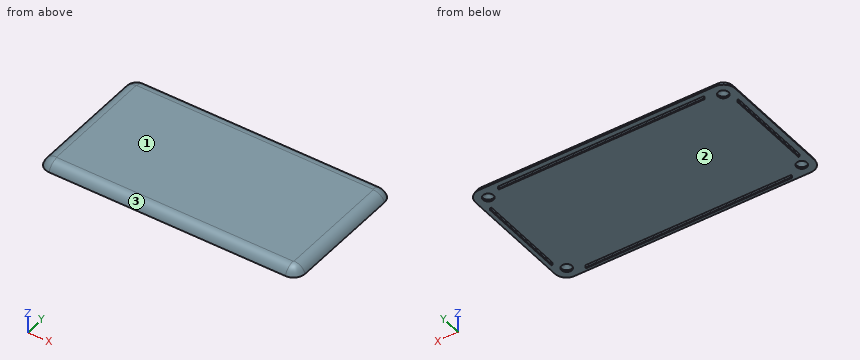
from build123d import *

# Parameters (mm, degrees)
F1_DEPTH     = 3.5
F5_D         = 4.473
F5_DEPTH     = 0.8
F5_TIP       = 1.3438247745
F6_T1_DEPTH  = 101
F6_T3_DEPTH  = 48.5
F6_T6_ANGLE  = 90
F6_T8_ANGLE  = 90
F6_T10_ANGLE = 90
F6_T12_ANGLE = 90
F8_W         = 0.5
F8_H         = 37.5
F8_W_2       = 88
F8_H_2       = 0.5
F9_DEPTH     = 1


# Not quite as in the source:
# - a fillet or chamfer that OpenCascade refuses, or shapes differently, is made with other operations: its cross-section is extruded or revolved along the edge and cut away or added


with BuildPart() as f1:
    # F0 (on Top) → F1 (new body)
    with BuildSketch(Plane.XY):
        with BuildLine():
            Line((-50.5, -29.25), (50.5, -29.25))
            ThreePointArc((50.5, -29.25), (54.0355339059, -27.7855339059), (55.5, -24.25))
            Line((55.5, -24.25), (55.5, 24.25))
            ThreePointArc((55.5, 24.25), (54.0355339059, 27.7855339059), (50.5, 29.25))
            Line((50.5, 29.25), (-50.5, 29.25))
            ThreePointArc((-50.5, 29.25), (-54.0355339059, 27.7855339059), (-55.5, 24.25))
            Line((-55.5, 24.25), (-55.5, -24.25))
            ThreePointArc((-55.5, -24.25), (-54.0355339059, -27.7855339059), (-50.5, -29.25))
        make_face()
    extrude(amount=F1_DEPTH)

    # F5
    with Locations(Plane(origin=(0, 0, 0), x_dir=(1, 0, 0), z_dir=(0, 0, -1))):
        with Locations((-50.2406740561, -23.9985361695), (-50.2495961264, 24.0030474961), (50.2488752827, 23.995583877), (50.2413948998, -24.0000952035)):
            Hole(F5_D / 2, depth=F5_DEPTH)
            with Locations((0, 0, -(F5_DEPTH + F5_TIP / 2))):  # 118° drill point
                Cone(0, F5_D / 2, F5_TIP, mode=Mode.SUBTRACT)

    # F6: fillet of radius 5 on 1 edges, made by hand

    # F6_s2 → F6_t1 (cut)
    with BuildSketch(Plane.YZ.offset(-50.5)):
        with BuildLine():
            ThreePointArc((-29.25, 0), (-27.4383438845, 2.5311288741), (-24.4803039929, 3.5))
            Line((-24.4803039929, 3.5), (-29.25, 3.5))
            Line((-29.25, 3.5), (-29.25, 0))
        make_face()
        with BuildLine():
            ThreePointArc((24.4803039929, 3.5), (27.4383438845, 2.5311288741), (29.25, 0))
            Line((29.25, 0), (29.25, 3.5))
            Line((29.25, 3.5), (24.4803039929, 3.5))
        make_face()
    extrude(amount=F6_T1_DEPTH, mode=Mode.SUBTRACT)

    # F6_s4 → F6_t3 (cut)
    with BuildSketch(Plane.XZ.offset(-24.25)):
        with BuildLine():
            ThreePointArc((50.7303039929, 3.5), (53.6883438845, 2.5311288741), (55.5, 0))
            Line((55.5, 0), (55.5, 3.5))
            Line((55.5, 3.5), (50.7303039929, 3.5))
        make_face()
        with BuildLine():
            ThreePointArc((-50.7303039929, 3.5), (-53.6883438845, 2.5311288741), (-55.5, 0))
            Line((-55.5, 0), (-55.5, 3.5))
            Line((-55.5, 3.5), (-50.7303039929, 3.5))
        make_face()
    extrude(amount=F6_T3_DEPTH, mode=Mode.SUBTRACT)

    # F6_s5 → F6_t6 (revolve, cut)
    with BuildSketch(Plane.XZ.offset(24.25)):
        with BuildLine():
            ThreePointArc((-55.5, 0), (-53.6883438845, 2.5311288741), (-50.7303039929, 3.5))
            Line((-50.7303039929, 3.5), (-55.5, 3.5))
            Line((-55.5, 3.5), (-55.5, 0))
        make_face()
    revolve(axis=Axis((-50.5, -24.25, 3.5), (0, 0, 1)), revolution_arc=F6_T6_ANGLE, mode=Mode.SUBTRACT)

    # F6_s7 → F6_t8 (revolve, cut)
    with BuildSketch(Plane.YZ.offset(50.5)):
        with BuildLine():
            ThreePointArc((-29.25, 0), (-27.4383438845, 2.5311288741), (-24.4803039929, 3.5))
            Line((-24.4803039929, 3.5), (-29.25, 3.5))
            Line((-29.25, 3.5), (-29.25, 0))
        make_face()
    revolve(axis=Axis((50.5, -24.25, 3.5), (0, 0, 1)), revolution_arc=F6_T8_ANGLE, mode=Mode.SUBTRACT)

    # F6_s9 → F6_t10 (revolve, cut)
    with BuildSketch(Plane.XZ.offset(-24.25)):
        with BuildLine():
            ThreePointArc((50.7303039929, 3.5), (53.6883438845, 2.5311288741), (55.5, 0))
            Line((55.5, 0), (55.5, 3.5))
            Line((55.5, 3.5), (50.7303039929, 3.5))
        make_face()
    revolve(axis=Axis((50.5, 24.25, 3.5), (0, 0, 1)), revolution_arc=F6_T10_ANGLE, mode=Mode.SUBTRACT)

    # F6_s11 → F6_t12 (revolve, cut)
    with BuildSketch(Plane.YZ.offset(-50.5)):
        with BuildLine():
            ThreePointArc((24.4803039929, 3.5), (27.4383438845, 2.5311288741), (29.25, 0))
            Line((29.25, 0), (29.25, 3.5))
            Line((29.25, 3.5), (24.4803039929, 3.5))
        make_face()
    revolve(axis=Axis((-50.5, 24.25, 3.5), (0, 0, 1)), revolution_arc=F6_T12_ANGLE, mode=Mode.SUBTRACT)

    # F8 (on Top) → F9 (join)
    with BuildSketch(Plane.XY):
        with Locations((-52.7812354267, 0)):
            Rectangle(F8_W, F8_H)
        with Locations((-0.0016481951, -26.7570052035)):
            Rectangle(F8_W_2, F8_H_2)
        with Locations((52.8098009527, 0)):
            Rectangle(F8_W, F8_H)
        with Locations((-0.0016481951, 26.78494009)):
            Rectangle(F8_W_2, F8_H_2)
    extrude(amount=-F9_DEPTH)


solid = f1.part
For this review, take the finished solid that the model builds, in its own axes (mm). Face numbers are marked on the shaded views. Round coordinates to 2 decimals unless told otherwise and drop trailing zeros. Write each loop counter-clockwise with the first axis right and the second up, starting at its lowest first coordinate (ties: lowest second). Pieces come first, ordered by that corner, then holes. Notation, with made-up numbers: (45, 66) - (83, 66) arc R16 cw to (83, 83) - close; hole circle Ø4 at (29.25, 80.5). An arc over 180 degrees is marked (long way). Write item = value, one per line. Start each with the question number.
1. Consider section B-B on x = 2. State the section outline as (y, z) points, plus the area to 3 significant figures.
2. Consider section C-C on x = 45.5. State the section outline as (y, z) points.
3. For pin 1 Ø2 at (x, z) = (22.5, 2.5) entering from -Y; pin 2 Ø0.5 at (x, z) = (-2, -0.5) entering from +Y; pin 3 Ø5 at (x, y) = (-24, -19) entering from -Z; pin 4 Ø1.1 at (y, z) = (7, -0.5) entering from +X, all flat-tipped, find the tip position at first contact; note any pin that passes through.
4. Draft analysis for pull direction Y (two halves, no side actions). For the marked faces 1, 2 and 3, state which applies: released by +Y, released by -Y, zero draft, split by the parting line, or undercut.
5. Wall thickness on L1, parallel to Y at x = 50, z = 1; L2, parallel to X at y = -11.5, z = -0.75; L3, parallel to Y at x = 31, z = -0.4: over which ranges is each line inside the solid? List them lowest first.
6. Consider section A-A on y = 13. State the section outline as (x, z) points, plus the area to 3 significant figures.
Evaluation:
q1.outline = (-29.25, 0) - (-27.01, 0) - (-27.01, -1) - (-26.51, -1) - (-26.51, 0) - (26.53, 0) - (26.53, -1) - (27.03, -1) - (27.03, 0) - (29.25, 0) arc R5 ccw to (24.48, 3.5) - (-24.48, 3.5) arc R5 ccw to start
q1.area = 197 mm2
q2.outline = (-29.25, 0) - (29.25, 0) arc R5 ccw to (24.48, 3.5) - (-24.48, 3.5) arc R5 ccw to start
q3.pin_1 = -28.48
q3.pin_2 = 27.03
q3.pin_3 = 0
q3.pin_4 = 55.5
q4.face_1 = zero draft
q4.face_2 = undercut
q4.face_3 = released by -Y
q5.L1 = -28.81 to -25.88, -22.11 to 22.11, 25.89 to 28.81
q5.L2 = -53.03 to -52.53, 52.56 to 53.06
q5.L3 = -27.01 to -26.51, 26.53 to 27.03
q6.outline = (-55.5, 0) - (-53.03, 0) - (-53.03, -1) - (-52.53, -1) - (-52.53, 0) - (52.56, 0) - (52.56, -1) - (53.06, -1) - (53.06, 0) - (55.5, 0) arc R5 ccw to (50.73, 3.5) - (-50.73, 3.5) arc R5 ccw to start
q6.area = 381 mm2
